from build123d import *

# Parameters (mm, degrees)
SKETCH1_W               = 50.8
SKETCH1_H               = 25.4
SKETCH1_W_2             = 44.45
SKETCH1_H_2             = 19.05
BOSS_EXTRUDE1_DEPTH     = 857.25
CUT_EXTRUDE1_DEPTH      = 860.129421275
CUT_EXTRUDE1_DEPTH_BACK = 860.129421275
SKETCH2_R               = 3.175
CUT_EXTRUDE2_DEPTH      = 860.129421275
CUT_EXTRUDE2_DEPTH_BACK = 860.129421275
SKETCH3_R               = 3.175


with BuildPart() as part:
    # Sketch1 → Boss-Extrude1 (new body)
    with BuildSketch(Plane.XY):
        with Locations((25.4, 12.7)):
            Rectangle(SKETCH1_W, SKETCH1_H)
        with Locations((25.4, 12.7)):
            Rectangle(SKETCH1_W_2, SKETCH1_H_2, mode=Mode.SUBTRACT)
    extrude(amount=BOSS_EXTRUDE1_DEPTH)

    # Sketch2 → Cut-Extrude1 (cut, two sides: drawn at the far end of the back side and taken through both)
    with BuildSketch(Plane(origin=(50.8, 0, 0), x_dir=(0, 0, -1), z_dir=(1, 0, 0)).offset(-CUT_EXTRUDE1_DEPTH_BACK)):
        with Locations((-88.9, 12.7)):
            Circle(SKETCH2_R)
        with Locations((-101.6, 12.7)):
            Circle(SKETCH2_R)
        with Locations((-114.3, 12.7)):
            Circle(SKETCH2_R)
    extrude(amount=CUT_EXTRUDE1_DEPTH + CUT_EXTRUDE1_DEPTH_BACK, mode=Mode.SUBTRACT)

    # Sketch3 → Cut-Extrude2 (cut, two sides: drawn at the far end of the back side and taken through both)
    with BuildSketch(Plane(origin=(0, 25.4, 0), x_dir=(1, 0, 0), z_dir=(0, 1, 0)).offset(-CUT_EXTRUDE2_DEPTH_BACK)):
        with Locations(Location((12.7, -31.75, 0), (0, 0, 270))):
            Circle(SKETCH3_R)
        with Locations(Location((25.4, -31.75, 0), (0, 0, 270))):
            Circle(SKETCH3_R)
        with Locations(Location((38.1, -31.75, 0), (0, 0, 270))):
            Circle(SKETCH3_R)
        with Locations(Location((25.4, -44.45, 0), (0, 0, 270))):
            Circle(SKETCH3_R)
        with Locations(Location((38.1, -44.45, 0), (0, 0, 270))):
            Circle(SKETCH3_R)
        with Locations(Location((25.4, -57.15, 0), (0, 0, 270))):
            Circle(SKETCH3_R)
        with Locations(Location((38.1, -57.15, 0), (0, 0, 270))):
            Circle(SKETCH3_R)
        with Locations(Location((12.7, -44.45, 0), (0, 0, 270))):
            Circle(SKETCH3_R)
        with Locations(Location((12.7, -57.15, 0), (0, 0, 270))):
            Circle(SKETCH3_R)
    extrude(amount=CUT_EXTRUDE2_DEPTH + CUT_EXTRUDE2_DEPTH_BACK, mode=Mode.SUBTRACT)


solid = part.part
Verification items for the finished model (mm, model axes). A direction names the side the tool comes from. Give positions to 0.01 mm unless a question says otherwise; leave off trailing zeros. Order: outer loops, then holes, each group sorted by start corner. A loop starts at its lowest first (then second) coordinate and runs counter-clockwise, first axis right, second up. Notation, with made-up numbers: M -9.75,-5.75 L 18.25,-5.75 A23 cw 18.25,30.25 Z; hole C -33.75,77.5 d5. An arc over 180 degrees is marked long. Use one line per item in the form item = value. Start each with the question number.
Q1. Access from +Z, -Z, +X, -X, +Y, -Y to the whole of each face (thin tool, end or side, straight path). Record for faces 5 (the flat face through (25, 22.225, 423)), 6 (the flat face through (25, 25.4, 423)).
Q2. Section check A-A (z = 241). Enter the section's corners in (x, y) (3 decimals), then the cut area to 3 significant figures.
Q3. Scan lines: line 1 along Z through (x, y) = (12.7, 0.75) (3 decimals); line 2 along Z through (x, y) = (49.3, 12.7) (3 decimals); line 3 along X through (y, z) = (0.65, 31.75) (3 decimals). Record each from-to range of solid material in increasing order. Write a range as [from, to].
Q4. Mould release check, pull along X, two halves, no side actions. Record for faces 1 (the flat face through (0, 13, 423)), 2 (the flat face through (50.8, 13, 423)), 3 (the flat face through (47.625, 13, 423)), 4 (the flat face through (3.175, 13, 423)): +X half, -X half, draft (parallel to the pull), parting line (faces both ways), or undercut.
Evaluation:
q1.face_5 = +Z, -Z
q1.face_6 = +Z, -Z, +X, -X, +Y
q2.outline = M 0,0 L 50.8,0 L 50.8,25.4 L 0,25.4 Z; hole M 3.175,3.175 L 47.625,3.175 L 47.625,22.225 L 3.175,22.225 Z
q2.area = 444 mm2
q3.line_1 = [0, 28.575], [34.925, 41.275], [47.625, 53.975], [60.325, 857.25]
q3.line_2 = [0, 85.725], [92.075, 98.425], [104.775, 111.125], [117.475, 857.25]
q3.line_3 = [0, 9.525], [15.875, 22.225], [28.575, 34.925], [41.275, 50.8]
q4.face_1 = -X half
q4.face_2 = +X half
q4.face_3 = undercut
q4.face_4 = undercut
